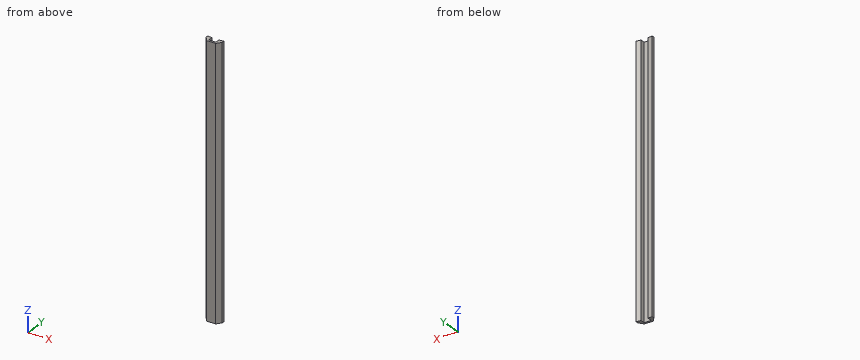
Autodesk Inventor part; units mm, degrees
ref_plane "YZ Plane" through (0, 0, 0) normal (1, 0, 0) x (0, 1, 0)
ref_plane "XZ Plane" through (0, 0, 0) normal (0, 1, 0) x (-1, 0, 0)
ref_plane "XY Plane" through (0, 0, 0) normal (0, 0, 1) x (1, 0, 0)
sketch "Sketch1" plane through (0, 0, 0) normal (0, 0, 1) x (1, 0, 0)
  line L0 (0, 0) -> (10.795, 0)
  line L1 (10.795, 0) -> (10.795, 4.7625)
  line L2 (0, 0) -> (0, 4.7625)
  arc A0 (0, 4.7625) -> (10.795, 4.7625) centre (5.3975, 55.2749) ccw
  dimension "d0" = 50.8
  dimension "d1" = 10.795
  dimension "d2" = 4.7625
extrude "Extrusion1" add sketch "Sketch1" along normal blind 177.8
sketch "Sketch2" plane through (0, 0, 177.8) normal (0, 0, 1) x (1, 0, 0)
  arc A0 (0, 4.7625) -> (10.795, 4.7625) centre (5.3975, 55.2749) ccw
  line L0 (3.0162, 4.5308) -> (7.7787, 4.5308)
  line L1 (7.7787, 4.5308) -> (7.7787, 1.3558)
  line L2 (7.7787, 1.3558) -> (3.0162, 1.3558)
  line L3 (3.0162, 1.3558) -> (3.0162, 4.5308)
  point P0 (0, 0)
  point P1 (5.3975, 4.5308)
  point P2 (5.3975, 4.4749)
  dimension "d5" = 4.7625
  dimension "d6" = 3.175
extrude "Extrusion2" cut sketch "Sketch2" against normal through all contours A0 L1 L2 L3
chamfer "Chamfer2" distance 3.175 distance2 2.286 1 edges at (0, 0, 88.9) measured on face at (0, 3.175, 118.5333)
chamfer "Chamfer3" distance 2.286 distance2 3.175 1 edges at (10.795, 0, 88.9) measured on face at (5.1223, 0, 59.2667)
properties part number "WireGuideToMiniSub" material "ABS Plastic"
CAD build for the part. Positions are in the model's coordinates, mm. Coordinates: 2 decimals unless noted, no trailing zeros. Write each loop counter-clockwise with the first axis right and the second up, starting at its lowest first coordinate (ties: lowest second). Pieces come first, ordered by that corner, then holes.
(1) Cut at B-B, the plane z = 28. List the corners of the cut face in (x, y) (1 decimal).
(2) Cut at A-A, the plane y = 2.25. List the corners of the cut face in (x, z), and give its area (3 significant figures).
(3) Flat gauge pin, fed straight in: pin 1 (4 mm diameter, centred on x = 5.5, z = 53.5, fed in from +Y). Where does the tip first touch, or does it go through?
(4) Cut at C-C, the plane x = 6. List the corners of the cut face in (y, z).
(5) Drill centre lines: probe 1 along X at (y, z) = (3.85, 90.5) (3 decimals); probe 2 along Y at (x, z) = (6.25, 20); probe 3 along X at (y, z) = (2.2, 96). Where is each one in solid material? Low to high.
Geometry says:
1. outline: (0, 3.2) - (2.3, 0) - (8.5, 0) - (10.8, 3.2) - (10.8, 4.8) arc R50.8 cw to (7.8, 4.5) - (7.8, 1.4) - (3, 1.4) - (3, 4.5) arc R50.8 cw to (0, 4.8) - close
2. outline: (0.67, 0) - (3.02, 0) - (3.02, 177.8) - (0.67, 177.8) - close; (7.78, 0) - (10.13, 0) - (10.13, 177.8) - (7.78, 177.8) - close
2. area: 836 mm2
3. pin 1: stops at y = 1.36
4. outline: (0, 0) - (1.36, 0) - (1.36, 177.8) - (0, 177.8) - close
5. probe 1: x = 0 to 3.016, 7.779 to 10.795
5. probe 2: y = 0 to 1.36
5. probe 3: x = 0.7 to 3.02, 7.78 to 10.09
